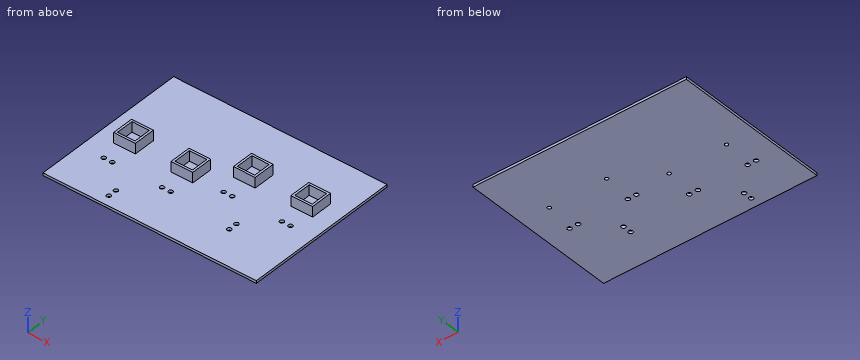
```python
from build123d import *

# Parameters (mm, degrees)
CROQUIS1_W              = 134
CROQUIS1_H              = 54
SALIENTE_EXTRUIR1_DEPTH = 3
CROQUIS2_W              = 25.3
CROQUIS2_H              = 25.3
CROQUIS2_W_2            = 20.3
CROQUIS2_H_2            = 20.3
SALIENTE_EXTRUIR2_DEPTH = 12
CROQUIS4_R              = 2
CORTAR_EXTRUIR1_DEPTH   = 12
CROQUIS5_W              = 115
CROQUIS5_H              = 30
SALIENTE_EXTRUIR3_DEPTH = 3
CROQUIS6_W              = 249
CROQUIS6_H              = 40
CROQUIS6_H_2            = 60
SALIENTE_EXTRUIR4_DEPTH = 3
CROQUIS8_R              = 2.5
CORTAR_EXTRUIR3_DEPTH   = 10


with BuildPart() as part:
    # Croquis1 → Saliente-Extruir1 (new body)
    with BuildSketch(Plane.XY):
        Rectangle(CROQUIS1_W, CROQUIS1_H)
    extrude(amount=SALIENTE_EXTRUIR1_DEPTH)

    # Croquis2 → Saliente-Extruir2 (add)
    # profile 1 of 2: a face of its own
    with BuildSketch(Plane.XY.offset(3)):
        with Locations((-33.5, 0)):
            Rectangle(CROQUIS2_W, CROQUIS2_H)
        with Locations((-33.5, 0)):
            Rectangle(CROQUIS2_W_2, CROQUIS2_H_2, mode=Mode.SUBTRACT)
    # profile 2 of 2: a face of its own
    with BuildSketch(Plane.XY.offset(3)):
        with Locations((33.5, 0)):
            Rectangle(CROQUIS2_W, CROQUIS2_H)
        with Locations((33.5, 0)):
            Rectangle(CROQUIS2_W_2, CROQUIS2_H_2, mode=Mode.SUBTRACT)
    extrude(amount=SALIENTE_EXTRUIR2_DEPTH)


with BuildPart() as body_2:
    # Sólido-Mover/Copiar1: copy of part
    add(part.part.moved(Location((115, 30, 0))))

    # Combinar1: union part
    add(part.part)

    # Croquis4 → Cortar-Extruir1 (cut)
    with BuildSketch(Plane.XY.offset(3)):
        with Locations((-33.5, 0)):
            Circle(CROQUIS4_R)
        with Locations((33.5, 0)):
            Circle(CROQUIS4_R)
        with Locations((81.5, 30)):
            Circle(CROQUIS4_R)
        with Locations((148.5, 30)):
            Circle(CROQUIS4_R)
    extrude(amount=-CORTAR_EXTRUIR1_DEPTH, mode=Mode.SUBTRACT)

    # Croquis5 → Saliente-Extruir3 (add)
    with BuildSketch(Plane.XY.offset(3)):
        with Locations((-9.5, 42)):
            Rectangle(CROQUIS5_W, CROQUIS5_H)
        with Locations((124.5, -12)):
            Rectangle(CROQUIS5_W, CROQUIS5_H)
    extrude(amount=-SALIENTE_EXTRUIR3_DEPTH)

    # Croquis6 → Saliente-Extruir4 (add)
    with BuildSketch(Plane.XY.offset(3)):
        with Locations((57.5, 77)):
            Rectangle(CROQUIS6_W, CROQUIS6_H)
        with Locations((57.5, -57)):
            Rectangle(CROQUIS6_W, CROQUIS6_H_2)
    extrude(amount=-SALIENTE_EXTRUIR4_DEPTH)

    # Croquis8 → Cortar-Extruir3 (cut)
    with BuildSketch(Plane.XY.offset(3)):
        with Locations((144, -5.15)):
            Circle(CROQUIS8_R)
        with Locations((154, -5.15)):
            Circle(CROQUIS8_R)
        with Locations((115, -34.15)):
            Circle(CROQUIS8_R)
        with Locations((115, -44.15)):
            Circle(CROQUIS8_R)
        with Locations(Location((76, -5.15, 0), (0, 0, 180))):
            Circle(CROQUIS8_R)
        with Locations(Location((86, -5.15, 0), (0, 0, 180))):
            Circle(CROQUIS8_R)
        with Locations((-29, -35.15)):
            Circle(CROQUIS8_R)
        with Locations((-39, -35.15)):
            Circle(CROQUIS8_R)
        with Locations((0, -65.15)):
            Circle(CROQUIS8_R)
        with Locations((0, -75.15)):
            Circle(CROQUIS8_R)
        with Locations(Location((39, -35.15, 0), (0, 0, 180))):
            Circle(CROQUIS8_R)
        with Locations(Location((29, -35.15, 0), (0, 0, 180))):
            Circle(CROQUIS8_R)
    extrude(amount=-CORTAR_EXTRUIR3_DEPTH, mode=Mode.SUBTRACT)


solid = body_2.part
```
Here's how the part is built. I have some questions about the finished solid (model axes, mm). Coordinates: 2 decimals unless noted, no trailing zeros. Order: outer loops, then holes, each group sorted by start corner. A loop starts at its lowest first (then second) coordinate and runs counter-clockwise, first axis right, second up.
1) Imagine slicing it at D-D on y = 62.5. List the corners of the cut face in (x, z) for me.
2) Imagine slicing it at A-A on z = 10. State how many separate pieces and enclosed holes the cut face has, and give its area (3 significant figures).
3) Imagine slicing it at B-B on x = 76. List the corners of the cut face in (y, z) for me, and give its area (3 significant figures).
4) Imagine slicing it at C-C on x = 0. List the corners of the cut face in (y, z) for me.
5) Will these pins go through, and if not, where does the flat tip stop? pin 1 (2 mm diameter, centred on x = 0, y = 17, fed in from -Z); pin 2 (6 mm diameter, centred on y = 33, z = 8, fed in from +X); pin 3 (3.5 mm diameter, centred on x = -27, z = 11.5, fed in from +Y); pin 4 (6 mm diameter, centred on x = 150.5, z = 8, fed in from +Y).
6) I need wall thicknesses on line 1 (X direction, y = 3, z = 14.75); line 2 (Y direction, x = 115, z = 1.8); line 3 (Z direction, x = -15, y = -29). Which ranges of each line are inside material? Lowest first, please.
Response values:
1. outline: (-67, 0) - (182, 0) - (182, 3) - (-67, 3) - close
2. separate pieces: 4
2. enclosed holes: 4
2. area: 912 mm2
3. outline: (-87, 0) - (-7.65, 0) - (-7.65, 3) - (-87, 3) - close; (-2.65, 0) - (97, 0) - (97, 3) - (42.65, 3) - (42.65, 15) - (40.15, 15) - (40.15, 3) - (19.85, 3) - (19.85, 15) - (17.35, 15) - (17.35, 3) - (-2.65, 3) - close
3. area: 597 mm2
4. outline: (-87, 0) - (-77.65, 0) - (-77.65, 3) - (-87, 3) - close; (-72.65, 0) - (-67.65, 0) - (-67.65, 3) - (-72.65, 3) - close; (-62.65, 0) - (97, 0) - (97, 3) - (-62.65, 3) - close
5. pin 1: stops at z = 0
5. pin 2: stops at x = 161.15
5. pin 3: stops at y = 12.65
5. pin 4: stops at y = 42.65
6. line 1: x = -46.15 to -43.65, -23.35 to -20.85, 20.85 to 23.35, 43.65 to 46.15
6. line 2: y = -87 to -46.65, -41.65 to -36.65, -31.65 to 97
6. line 3: z = 0 to 3
